CAD build for the part. Positions are in the model's coordinates, mm. A direction names the side the tool comes from. Give positions to 0.01 mm unless a question says otherwise; leave off trailing zeros. Write each loop counter-clockwise with the first axis right and the second up, starting at its lowest first coordinate (ties: lowest second). Pieces come first, ordered by that corner, then holes. Notation, with made-up numbers: (-27, 51.5) - (-11, 51.5) arc R16 cw to (-11, 62.5) - close; hole circle Ø11 at (-36.5, 42). An arc over 180 degrees is marked (long way). Answer as a JSON object with one key per item and string values.
from build123d import *

# Parameters (mm, degrees)
CUT_EXTRUDE_START   = -2
SKETCH_4_R          = 9
CUT_EXTRUDE_1_DEPTH = 2
EXTRUDE_START       = -12
SKETCH_5_R          = 8
SKETCH_5_R_2        = 5.5
EXTRUDE_1_DEPTH     = 12
CHAMFER_1_SIZE      = 0.5


with BuildPart() as part:
    # Эскиз1 → Повернуть1 (revolve)
    with BuildSketch(Plane.XY, mode=Mode.PRIVATE) as revolve_1_sk:
        Polygon((0, 5.5), (20, 5.5), (20, 9), (18, 9), (18, 7), (0, 7), align=None)
    revolve(revolve_1_sk.sketch.rotate(Axis((0, 0, 0), (1, 0, 0)), 90), axis=Axis((0, 0, 0), (1, 0, 0)))

    # Эскиз4 → Вырез-Вытянуть1 (cut)
    with BuildSketch(Plane(origin=(20, 0, 0), x_dir=(0, 0, -1), z_dir=(1, 0, 0)).offset(CUT_EXTRUDE_START)):
        Circle(SKETCH_4_R)
    extrude(amount=CUT_EXTRUDE_1_DEPTH, mode=Mode.SUBTRACT)

    # Эскиз5 → Бобышка-Вытянуть1 (add)
    with BuildSketch(Plane.ZY.offset(EXTRUDE_START)):
        Circle(SKETCH_5_R)
        Circle(SKETCH_5_R_2, mode=Mode.SUBTRACT)
    extrude(amount=EXTRUDE_1_DEPTH)

    # Фаска1
    chamfer_1_edges = [part.edges().sort_by_distance(p)[0] for p in [
        (18, 0, -7),
        (12, 0, -8),
        (0, 0, -8),
    ]]
    chamfer(chamfer_1_edges, length=CHAMFER_1_SIZE)


solid = part.part
Item 1: Mould opens along Y. For faces 1 (the cylindrical face through (9.13, 5.37, -1.19)), 2 (the cylindrical face through (6.08, -7.81, -1.73)), 3 (the flat face through (18, 3, 5)) say: +Y half, -Y half, draft (parallel to the pull), parting line (faces both ways), or undercut.
Entries:
{"face 1": "undercut", "face 2": "parting line", "face 3": "draft"}
Item 2: Which spindle directions (+Z, -Z, +X, -X, +Y, -Y) get a long thin tool onto all of the face, cutting with end or side? Do faces 4 (the cylindrical face through (14.71, 6.21, 3.23)), 5 (the flat face through (0, 4, -4)). Say none if no direction does.
Entries:
{"face 4": "+X", "face 5": "+Z, -Z, -X, +Y, -Y"}
Item 3: Cut at A-A (z = 0). Give the cut face in (x, y), and give its area (4 significant figures).
Entries:
{"outline": "(0, -7.5) - (0.5, -8) - (11.5, -8) - (12, -7.5) - (12, -7) - (17.5, -7) - (18, -6.5) - (18, -5.5) - (0, -5.5) - close; (0, 5.5) - (18, 5.5) - (18, 6.5) - (17.5, 7) - (12, 7) - (12, 7.5) - (11.5, 8) - (0.5, 8) - (0, 7.5) - close", "area": "77.25 mm2"}
Item 4: Probe line 1 (Y direction, x = 16.75, z = 0.25); line 2 (Y direction, x = 6.75, z = 0); line 3 (Z direction, x = 15.25, y = 0.75). List the from-to ranges inside material, lowest first. Write a range as from..to.
Entries:
{"line 1": "-7..-5.49, 5.49..7", "line 2": "-8..-5.5, 5.5..8", "line 3": "-6.96..-5.45, 5.45..6.96"}
Item 5: Flat gauge pins, fed straight in: P1, Ø1.5, axis at x = 10.5, y = -4.5, coming from the -Z side; P2, Ø8, axis at x = 6.5, z = 5, coming from the +Y side; P3, Ø1.5, axis at x = 15.5, z = -0.5, coming from the +Y side. Where does each tip first touch, or does it go through?
Entries:
{"P1": "z = -7.07", "P2": "y = 7.94", "P3": "y = 7"}
Item 6: Cut at C-C (x = 2.5). Give the cut face in (y, z).
Entries:
{"outline": "circle Ø16 at (0, 0); hole circle Ø11 at (0, 0)"}
Item 7: Cut at D-D (x = 14.5). Give the cut face in (y, z), and give its area (3 significant figures).
Entries:
{"outline": "circle Ø14 at (0, 0); hole circle Ø11 at (0, 0)", "area": "58.9 mm2"}
